Input: part model. Units: mm. Frame: model coordinates. Give positions to 0.01 mm unless a question says otherwise; leave off trailing zeros. Loops run counter-clockwise (first coordinate to the right, second up) from the corner with the lowest first, then second, coordinate; pieces in that order, holes last. Notation, with made-up numbers: (14, -31.75) - (71, -31.75) arc R21 ccw to (71, -9.75) - close; hole circle Ø10 at (-15.5, -30). An arc over 180 degrees is marked (long way). Answer as a JSON object with one key per item and string values.
from build123d import *

# Parameters (mm, degrees)
BOSS_EXTRUDE1_DEPTH = 5
SKETCH3_R           = 1.5
CUT_EXTRUDE1_DEPTH  = 5


with BuildPart() as part:
    # Sketch2 → Boss-Extrude1 (new body)
    with BuildSketch(Plane.XY):
        with BuildLine():
            Line((0, 15), (50, 15))
            ThreePointArc((50, 15), (65, 0), (50, -15))
            Line((50, -15), (0, -15))
            ThreePointArc((0, -15), (-15, 0), (0, 15))
        make_face()
    extrude(amount=BOSS_EXTRUDE1_DEPTH)

    # Sketch3 → Cut-Extrude1 (cut)
    with BuildSketch(Plane(origin=(0, 0, 0), x_dir=(-1, 0, 0), z_dir=(0, 0, -1))):
        with Locations((-50, 0)):
            Circle(SKETCH3_R)
        Circle(SKETCH3_R)
    extrude(amount=-CUT_EXTRUDE1_DEPTH, mode=Mode.SUBTRACT)


solid = part.part
Item 1: Cut plane C-C (x = 59). Return loops of the section in (y, z).
Geometry check:
{"outline": "(-12, 0) - (12, 0) - (12, 5) - (-12, 5) - close"}
Item 2: Mould query, pull axis Y, two halves, no side actions, for faces 1 (the face through (25, 15, 2)), 2 (the face through (26, 0, 0)), 3 (the face through (1.5, 0.07, 2.46)), 4 (the face through (25, -15, 2)). Classes: released by +Y, released by -Y, zero draft, split by the parting line, or undercut.
Geometry check:
{"face 1": "released by +Y", "face 2": "zero draft", "face 3": "undercut", "face 4": "released by -Y"}
Item 3: Cut plane B-B (z = 2.2). Return loops of the section in (x, y).
Geometry check:
{"outline": "(0, -15) - (50, -15) arc R15 ccw to (50, 15) - (0, 15) arc R15 ccw to start; hole circle Ø3 at (0, 0); hole circle Ø3 at (50, 0)"}
Item 4: Cut plane D-D (y = -12). Return loops of the section in (x, z).
Geometry check:
{"outline": "(-9, 0) - (59, 0) - (59, 5) - (-9, 5) - close"}
Item 5: Contact query for flat-ended pins moving along their axis: P1, Ø3, axis at y = 9.5, z = 4.5, coming from the -X side; P2, Ø2.5, axis at x = 50, y = 0, coming from the +Z side; P3, Ø2, axis at y = 3.5, z = 1, coming from the +X side; P4, Ø2, axis at y = -3.5, z = 1, coming from the -X side. Output: stop coordinate, or through.
Geometry check:
{"P1": "stops at x = -12.69", "P2": "passes through", "P3": "stops at x = 64.79", "P4": "stops at x = -14.79"}
Item 6: Material intervals for line 1 (X direction, y = 1, z = 3.8); line 2 (Y direction, x = 0, z = 2); line 3 (X direction, y = 11.5, z = 0.3), sorted ascending. Write a range as [from, to].
Geometry check:
{"line 1": "x = [-14.97, -1.12], [1.12, 48.88], [51.12, 64.97]", "line 2": "y = [-15, -1.5], [1.5, 15]", "line 3": "x = [-9.63, 59.63]"}
Item 7: Cut plane A-A (y = 0). Return loops of the section in (x, z), then the cut area to 3 significant figures.
Geometry check:
{"outline": "(-15, 0) - (-1.5, 0) - (-1.5, 5) - (-15, 5) - close; (1.5, 0) - (48.5, 0) - (48.5, 5) - (1.5, 5) - close; (51.5, 0) - (65, 0) - (65, 5) - (51.5, 5) - close", "area": "370 mm2"}
